from build123d import *

# Parameters (mm, degrees)
SKETCH1_R           = 1.11125
BOSS_EXTRUDE1_DEPTH = 3.937
SKETCH2_R           = 1.27
CUT_EXTRUDE1_DEPTH  = 37.36946133


with BuildPart() as part:
    # Sketch1 → Boss-Extrude1 (new body)
    with BuildSketch(Plane.XY):
        with BuildLine():
            Line((-7.3406, 30.988), (-7.3406, 5.92501279))
            ThreePointArc((-7.3406, 5.92501279), (-7.122958425, 3.583917287), (-6.477493204, 1.323061108))
            ThreePointArc((-6.477493204, 1.323061108), (-9.8806, -3.65125), (-13.283706796, 1.323061108))
            ThreePointArc((-13.283706796, 1.323061108), (-12.638241575, 3.583917287), (-12.4206, 5.92501279))
            Line((-12.4206, 5.92501279), (-12.4206, 30.988))
            ThreePointArc((-12.4206, 30.988), (-9.8806, 33.528), (-7.3406, 30.988))
        make_face()
        with Locations(Location((-9.8806, 0, 0), (0, 0, 180))):
            Circle(SKETCH1_R, mode=Mode.SUBTRACT)
    extrude(amount=BOSS_EXTRUDE1_DEPTH)

    # Sketch2 → Cut-Extrude1 (cut, through all)
    with BuildSketch(Plane(origin=(0, 0, 0), x_dir=(-1, 0, 0), z_dir=(0, 0, -1))):
        with Locations((9.8806, 18.456506395)):
            Circle(SKETCH2_R)
    extrude(amount=-CUT_EXTRUDE1_DEPTH, mode=Mode.SUBTRACT)


solid = part.part
Work out the finished part from the listing and answer in its coordinate system (mm). A direction names the side the tool comes from. Round coordinates to 2 decimals unless told otherwise and drop trailing zeros. Loops run counter-clockwise (first coordinate to the right, second up) from the corner with the lowest first, then second, coordinate; pieces in that order, holes last. Notation, with made-up numbers: M 70,-21.5 L 95,-21.5 A22 cw 95,10.5 Z; hole C 72.5,89 d9. An arc over 180 degrees is marked long. One line per question, with ' | ' between items. Start each with the question number.
(1) A cutting plane is placed at C-C on y = 26.5. Write down the section's boundary in (x, z).
(2) Flat-ended cylindrical pins translate along their axes: pin 1 Ø2 at (y, z) = (16.5, 2.5) entering from -X; pin 2 Ø3 at (x, y) = (-11.5, 18.5) entering from -Z; pin 3 Ø1.5 at (y, z) = (2.5, 0.5) entering from -X; pin 4 Ø1.8 at (x, y) = (-9.88, 0) entering from +Z. Find the tip coordinate at first contact, or state that the pin passes through.
(3) A tool of negligible diameter and unlimited length cuts with its end or side. For faces 1 (the face through (-8.94, 19.31, 1.94)), 2 (the face through (-7.341, 19, 2)), from which of +Z, -Z, +X, -X, +Y, -Y can it reach the whole face along a straight path? Write none if from no direction.
(4) A cutting plane is placed at D-D on x = -8. Write down the section's boundary in (y, z).
(5) A cutting plane is placed at B-B on x = -10. Write down the section's boundary in (y, z).
(6) Find the intervals of material crossed by line 1 (Y direction, x = -9.75, z = 2.85); line 2 (Y direction, x = -10.75, z = 3.15); line 3 (X direction, y = 21, z = 3), in increasing order.
(7) For a pull along X with two mould halves and no side action, classify faces 3 (the face through (-9.78, -3.65, 1.94)), 4 (the face through (-8.77, -0.05, 1.94)), 5 (the face through (-10, 15, 3.937)), 6 (the face through (-12.421, 18, 2)) as released by +X, released by -X, zero draft, split by the parting line, or undercut.
(8) A cutting plane is placed at A-A on y = 0. Write down the section's boundary in (x, z), plus the area to 3 significant figures.
Geometry check:
1) outline: M -12.42,0 L -7.34,0 L -7.34,3.94 L -12.42,3.94 Z
2) pin 1: stops at x = -12.42 | pin 2: stops at z = 0 | pin 3: stops at x = -13.13 | pin 4: passes through
3) face 1: +Z, -Z | face 2: +Z, -Z, +X, +Y
4) outline: M -3.13,0 L 32.7,0 L 32.7,3.94 L -3.13,3.94 Z
5) outline: M -3.65,0 L -1.1,0 L -1.1,3.94 L -3.65,3.94 Z; M 1.1,0 L 17.19,0 L 17.19,3.94 L 1.1,3.94 Z; M 19.72,0 L 33.53,0 L 33.53,3.94 L 19.72,3.94 Z
6) line 1: y = -3.65 to -1.1, 1.1 to 17.19, 19.72 to 33.52 | line 2: y = -3.55 to -0.69, 0.69 to 17.53, 19.38 to 33.37 | line 3: x = -12.42 to -7.34
7) face 3: split by the parting line | face 4: undercut | face 5: zero draft | face 6: released by -X
8) outline: M -13.53,0 L -10.99,0 L -10.99,3.94 L -13.53,3.94 Z; M -8.77,0 L -6.23,0 L -6.23,3.94 L -8.77,3.94 Z | area: 20.0 mm²
